Model file for the job. Use its own axes, mm. A direction names the side the tool comes from. Coordinates: 2 decimals unless noted, no trailing zeros. Order: outer loops, then holes, each group sorted by start corner. A loop starts at its lowest first (then second) coordinate and runs counter-clockwise, first axis right, second up. Notation, with made-up numbers: M 30,26 L 53,26 A25 ccw 53,64 Z; hole C -35,23.5 d9. An arc over 180 degrees is marked long. Return JSON: item names as keys, results as strings.
```python
from build123d import *

# Parameters (mm, degrees)
SKIZZE1_W                       = 300
SKIZZE1_H                       = 75
LINEAR_AUSTRAGEN1_DEPTH         = 10
SKIZZE2_W                       = 100
SKIZZE2_H                       = 60
SCHNITT_LINEAR_AUSTRAGEN1_DEPTH = 10
VERRUNDUNG1_R                   = 3
SKIZZE4_W                       = 10
SKIZZE4_H                       = 30
SCHNITT_LINEAR_AUSTRAGEN2_DEPTH = 30


with BuildPart() as part:
    # Skizze1 → Linear austragen1 (new body)
    with BuildSketch(Plane.XY):
        with Locations((0, -112.5)):
            Rectangle(SKIZZE1_W, SKIZZE1_H)
    extrude(amount=LINEAR_AUSTRAGEN1_DEPTH)

    # Skizze2 → Schnitt-Linear austragen1 (cut)
    with BuildSketch(Plane.XY.offset(10)):
        with Locations((0, -110)):
            Rectangle(SKIZZE2_W, SKIZZE2_H)
    extrude(amount=-SCHNITT_LINEAR_AUSTRAGEN1_DEPTH, mode=Mode.SUBTRACT)

    # Verrundung1
    verrundung1_edges = [part.edges().sort_by_distance(p)[0] for p in [
        (50, -80, 5),
        (50, -140, 5),
        (-50, -140, 5),
        (-50, -80, 5),
    ]]
    fillet(verrundung1_edges, radius=VERRUNDUNG1_R)

    # Skizze4 → Schnitt-Linear austragen2 (cut)
    with BuildSketch(Plane(origin=(150, 0, 0), x_dir=(0, 0, -1), z_dir=(1, 0, 0))):
        with Locations((-5, -135)):
            Rectangle(SKIZZE4_W, SKIZZE4_H)
    schnitt_linear_austragen2 = extrude(amount=-SCHNITT_LINEAR_AUSTRAGEN2_DEPTH, mode=Mode.SUBTRACT)

    # Spiegeln1: Schnitt-Linear austragen2 across plane
    add(schnitt_linear_austragen2.mirror(Plane(origin=(0, 0, 0), x_dir=(0, 0, 1), z_dir=(1, 0, 0))), mode=Mode.SUBTRACT)


solid = part.part
```
Item 1: Saw through at C-C (z = 8). Write the cut outline in (x, y), and give its area (3 significant figures).
Check result:
{"outline": "M -150,-120 L -120,-120 L -120,-150 L 120,-150 L 120,-120 L 150,-120 L 150,-75 L -150,-75 Z; hole M -50,-137 A3 ccw -47,-140 L 47,-140 A3 ccw 50,-137 L 50,-83 A3 ccw 47,-80 L -47,-80 A3 ccw -50,-83 Z", "area": "14,700 mm2"}
Item 2: Saw through at D-D (x = -130.5). Write the cut outline in (y, z).
Check result:
{"outline": "M -120,0 L -75,0 L -75,10 L -120,10 Z"}
Item 3: Pull direction X, two halves, no side cores. Call faces 6 (the flat face through (-2, -79, 0)), 7 (the flat face through (50, -110, 5)), 8 (the flat face through (-120, -135, 5)): +X half, -X half, draft (parallel to the pull), parting line (faces both ways), or undercut.
Check result:
{"face 6": "draft", "face 7": "undercut", "face 8": "-X half"}
Item 4: Saw through at A-A (y = -93). Write the cut outline in (x, z).
Check result:
{"outline": "M -150,0 L -50,0 L -50,10 L -150,10 Z; M 50,0 L 150,0 L 150,10 L 50,10 Z"}
Item 5: Drop flat-ended pins along their axis: pin 1 Ø3 at (y, z) = (-139, 7) entering from -X; pin 2 Ø1 at (x, y) = (-22, -138) entering from -Z. Give the stop position or say it passes through.
Check result:
{"pin 1": "stops at x = -120", "pin 2": "passes through"}
Item 6: 3-axis set-ups, long thin cutter, end or side, ignore diameter. For faces 1 (the flat face through (-1, -140, 5)), 2 (the flat face through (150, -98, 5)), 3 (the flat face through (-135, -120, 5)), 4 (the flat face through (-2, -79, 10)), 5 (the flat face through (135, -120, 5)): which of +Z, -Z, +X, -X, +Y, -Y reach the whole face in a straight line?
Check result:
{"face 1": "+Z, -Z", "face 2": "+Z, -Z, +X, +Y, -Y", "face 3": "+Z, -Z, -X, -Y", "face 4": "+Z, +X, -X, +Y, -Y", "face 5": "+Z, -Z, +X, -Y"}
Item 7: Saw through at B-B (x = -29.5). Write the cut outline in (y, z), and give its area (3 significant figures).
Check result:
{"outline": "M -150,0 L -140,0 L -140,10 L -150,10 Z; M -80,0 L -75,0 L -75,10 L -80,10 Z", "area": "150 mm2"}
Item 8: Wall check: line 1 (Y direction, x = -1, z = 8); line 2 (X direction, y = -137, z = 4.75); line 3 (X direction, y = -95, z = 9.5). Give the ranges that are in metal, low to high.
Check result:
{"line 1": "y = -150 to -140, -80 to -75", "line 2": "x = -120 to -50, 50 to 120", "line 3": "x = -150 to -50, 50 to 150"}
